Drawing for the job (mm, zero at the part's lowest x, y, z). A direction names the side the tool comes from. Give positions to 0.01 mm unless a question says otherwise; leave off trailing zeros. Order: outer loops, then holes, each group sorted by start corner. A loop starts at its lowest first (then second) coordinate and runs counter-clockwise, first axis right, second up. Notation, with made-up numbers: (13, 21) - (27, 21) arc R20 ccw to (27, 42) - close; hole circle Ø10 at (28, 74.25). An arc over 180 degrees is marked (long way). Use a Markdown table: item, result. Add a question column.
(1) Which spindle directions (+Z, -Z, +X, -X, +Y, -Y) get a long thin tool onto all of the face, cutting with end or side? Do the marked faces 1, 2 and 3. Say none if no direction does.
(2) Mould opens along Y. For the marked faces 4, 5, 6 and 7 say: +Y half, -Y half, draft (parallel to the pull), parting line (faces both ways), or undercut.
(3) Wall check: line 1 (Y direction, x = 21.5, z = 9); line 2 (Z direction, x = 27, y = 51); line 3 (X direction, y = 32.5, z = 5). Give the ranges that are in metal, low to high.
(4) Slice it at C-C (z = 4.5). Write the cut outline in (x, y).
(5) Slice it at B-B (x = 30). Write the cut outline in (y, z).
(6) Slice it at D-D (y = 51). Write the cut outline in (x, z), then the cut area to 3 significant figures.
(7) Slice it at A-A (y = 11). Write the cut outline in (x, z).
(8) Flat gauge pins, fed straight in: pin 1 (6 mm diameter, centred on y = 26, z = 8, fed in from -X); pin 2 (4.5 mm diameter, centred on x = 21, z = 6.5, fed in from -Y); pin 3 (1 mm diameter, centred on y = 31, z = 9, fed in from +X). Where does each tip first touch, or does it go through?
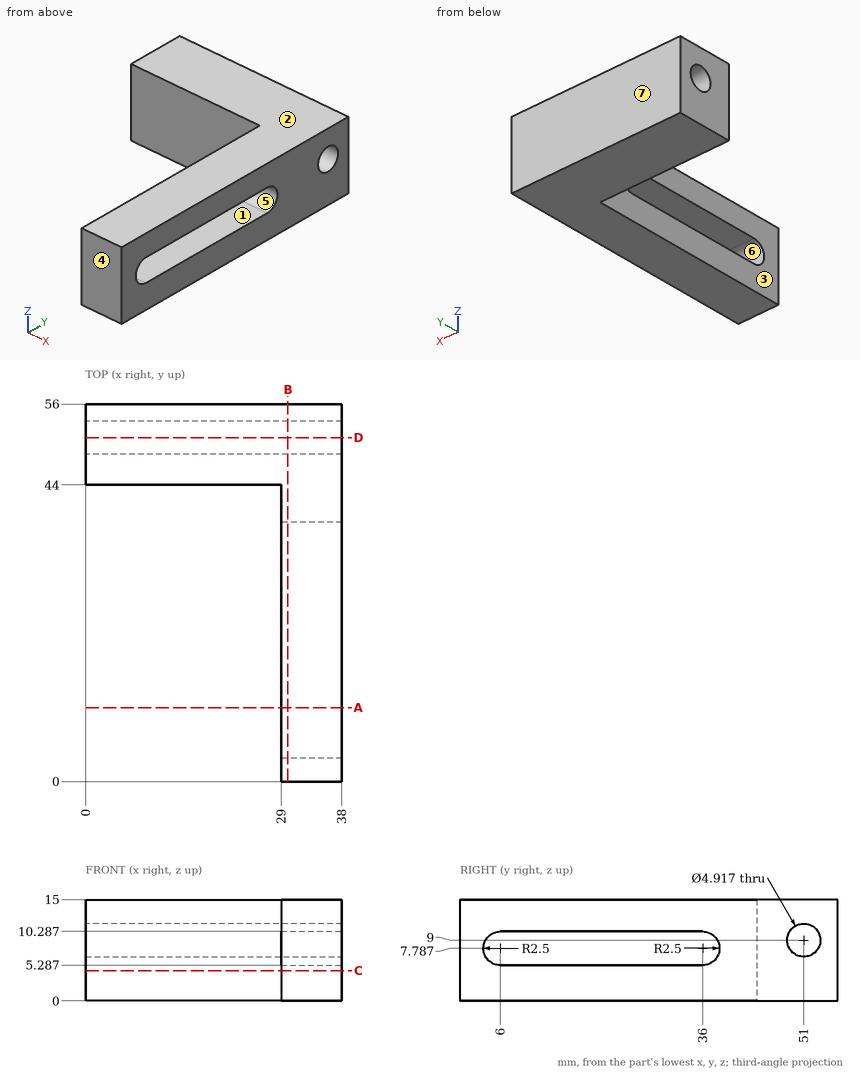
Solution:
| question | item | result |
|---|---|---|
| 1 | face 1 | +X, -X |
| 1 | face 2 | +Z, +X, -X, +Y, -Y |
| 1 | face 3 | +Z, -Z, -X, -Y |
| 2 | face 4 | -Y half |
| 2 | face 5 | undercut |
| 2 | face 6 | undercut |
| 2 | face 7 | +Y half |
| 3 | line 1 | 44 to 48.54, 53.46 to 56 |
| 3 | line 2 | 0 to 6.54, 11.46 to 15 |
| 3 | line 3 | 29 to 38 |
| 4 | outline | (0, 44) - (29, 44) - (29, 0) - (38, 0) - (38, 56) - (0, 56) - close |
| 5 | outline | (0, 0) - (56, 0) - (56, 15) - (0, 15) - close; hole (6, 5.29) - (36, 5.29) arc R2.5 ccw to (36, 10.29) - (6, 10.29) arc R2.5 ccw to start; hole circle Ø4.92 at (51, 9) |
| 6 | outline | (0, 0) - (38, 0) - (38, 6.54) - (0, 6.54) - close; (0, 11.46) - (38, 11.46) - (38, 15) - (0, 15) - close |
| 6 | area | 383 mm2 |
| 7 | outline | (29, 0) - (38, 0) - (38, 5.29) - (29, 5.29) - close; (29, 10.29) - (38, 10.29) - (38, 15) - (29, 15) - close |
| 8 | pin 1 | x = 29 |
| 8 | pin 2 | y = 44 |
| 8 | pin 3 | through |
